from build123d import *

# Parameters (mm, degrees)
SKETCH1_W                = 100
SKETCH1_H                = 140
SKETCH1_R                = 7.5
SKETCH1_R_2              = 2
SKETCH1_R_3              = 1.5
BOSS_EXTRUDE1_DEPTH      = 5
F_3_0_3_DIAMETER_HOLE1_D = 3


with BuildPart() as part:
    # Sketch1 → Boss-Extrude1 (new body)
    with BuildSketch(Plane(origin=(0, 0, 0), x_dir=(1, 0, 0), z_dir=(0, 1, 0))):
        Rectangle(SKETCH1_W, SKETCH1_H)
        with Locations(Location((-15, 0, 0), (0, 0, 270))):
            Circle(SKETCH1_R, mode=Mode.SUBTRACT)
        with Locations(Location((20, 0, 0), (0, 0, 270))):
            Circle(SKETCH1_R_2, mode=Mode.SUBTRACT)
        with Locations(Location((20, -17.5, 0), (0, 0, 270))):
            Circle(SKETCH1_R_3, mode=Mode.SUBTRACT)
        with Locations(Location((20, 17.5, 0), (0, 0, 270))):
            Circle(SKETCH1_R_3, mode=Mode.SUBTRACT)
    extrude(amount=BOSS_EXTRUDE1_DEPTH)

    # 3.0 _3_ Diameter Hole1 (through all)
    with Locations(Plane(origin=(0, 5, 0), x_dir=(-1, 0, 0), z_dir=(0, 1, 0))):
        with Locations((-42, 60), (42, 60), (42, -60), (-42, -60)):
            Hole(F_3_0_3_DIAMETER_HOLE1_D / 2)


solid = part.part
The model under review builds one solid part; all positions refer to its coordinate system, in mm. Round coordinates to 2 decimals unless told otherwise and drop trailing zeros. Loops run counter-clockwise (first coordinate to the right, second up) from the corner with the lowest first, then second, coordinate; pieces in that order, holes last. Notation, with made-up numbers: (34.25, 21.25) -> (64.25, 21.25) arc R24 ccw to (64.25, 33.25) -> close; hole circle Ø7 at (78.25, 21). An arc over 180 degrees is marked (long way). Write item = value, one per line. Start each with the question number.
Item 1: Take a section at D-D on z = 0. Give the boundary of the cut face in (x, y), plus the area to 3 significant figures.
Item 2: Take a section at A-A on x = 42. Give the boundary of the cut face in (y, z).
Item 3: Insertion check: pin 1 (3.5 mm diameter, centred on x = 20, z = 17.5, fed in from -Y). The pin has a flat end and moves straight along its axis. Give the tip position at first contact, or say it passes through.
Item 4: To check wall thickness, follow L1, parallel to Z at x = 42, y = 1; L2, parallel to X at y = 2.65, z = -17.5; L3, parallel to X at y = 0.7, z = -61. State the ranges of each line that lie inside material, in increasing order.
Item 5: Take a section at C-C on x = 20. Give the boundary of the cut face in (y, z), plus the area to 3 significant figures.
Item 6: Take a section at B-B on y = 1.55. Count the separate pieces of the cut face and the enclosed holes in it, plus the area to 3 significant figures.
Item 7: Mouldability with a two-part tool opening along X and no side actions: class faces 1 (the cylindrical face through (22, 2, 0)), 2 (the flat face through (50, 2, 1)), 3 (the cylindrical face through (-43.11, 2.47, 61.01)), 4 (the flat face through (-1, 5, -1)) as released by +X, released by -X, zero draft, split by the parting line, or undercut.
Result:
q1.outline = (-50, 0) -> (-22.5, 0) -> (-22.5, 5) -> (-50, 5) -> close; (-7.5, 0) -> (18, 0) -> (18, 5) -> (-7.5, 5) -> close; (22, 0) -> (50, 0) -> (50, 5) -> (22, 5) -> close
q1.area = 405 mm²
q2.outline = (0, -70) -> (5, -70) -> (5, -61.5) -> (0, -61.5) -> close; (0, -58.5) -> (5, -58.5) -> (5, 58.5) -> (0, 58.5) -> close; (0, 61.5) -> (5, 61.5) -> (5, 70) -> (0, 70) -> close
q3.pin_1 = 0
q4.L1 = -70 to -61.5, -58.5 to 58.5, 61.5 to 70
q4.L2 = -50 to 18.5, 21.5 to 50
q4.L3 = -50 to -43.12, -40.88 to 40.88, 43.12 to 50
q5.outline = (0, -70) -> (5, -70) -> (5, -19) -> (0, -19) -> close; (0, -16) -> (5, -16) -> (5, -2) -> (0, -2) -> close; (0, 2) -> (5, 2) -> (5, 16) -> (0, 16) -> close; (0, 19) -> (5, 19) -> (5, 70) -> (0, 70) -> close
q5.area = 650 mm²
q6.separate_pieces = 1
q6.enclosed_holes = 8
q6.area = 13,800 mm²
q7.face_1 = undercut
q7.face_2 = released by +X
q7.face_3 = undercut
q7.face_4 = zero draft
